The drawing under review shows one solid part. Ordinate dimensions are in mm from its lowest x, y, z. Coordinates: 2 decimals unless noted, no trailing zeros. Write each loop counter-clockwise with the first axis right and the second up, starting at its lowest first coordinate (ties: lowest second). Pieces come first, ordered by that corner, then holes.
1) We need section C-C on z = 55. Write out the cut boundary in (x, y), then the cut area to 3 significant figures.
2) We need section B-B on y = 4.1. Give the number of separate pieces and of enclosed holes in the cut face, then the cut area to 3 significant figures.
3) To check wall thickness, follow line 1 along Z through (x, y) = (27, 3.6); line 2 along Z through (x, y) = (52, 3); line 3 along X through (y, z) = (4.85, 52.5). State the ranges of each line that lie inside material, in increasing order.
4) Insertion check: P1, Ø10, axis at x = 12.5, z = 57.5, coming from the -Y side; P2, Ø2, axis at x = 8.5, y = 3.5, coming from the +Z side. Each pin has a flat end and moves straight along its axis. Give the tip position at first contact, or say it passes through.
5) We need section A-A on x = 27. Write out the cut boundary in (y, z).
6) We need section D-D on z = 22.5. Write out the cut boundary in (x, y), then the cut area to 3 significant figures.
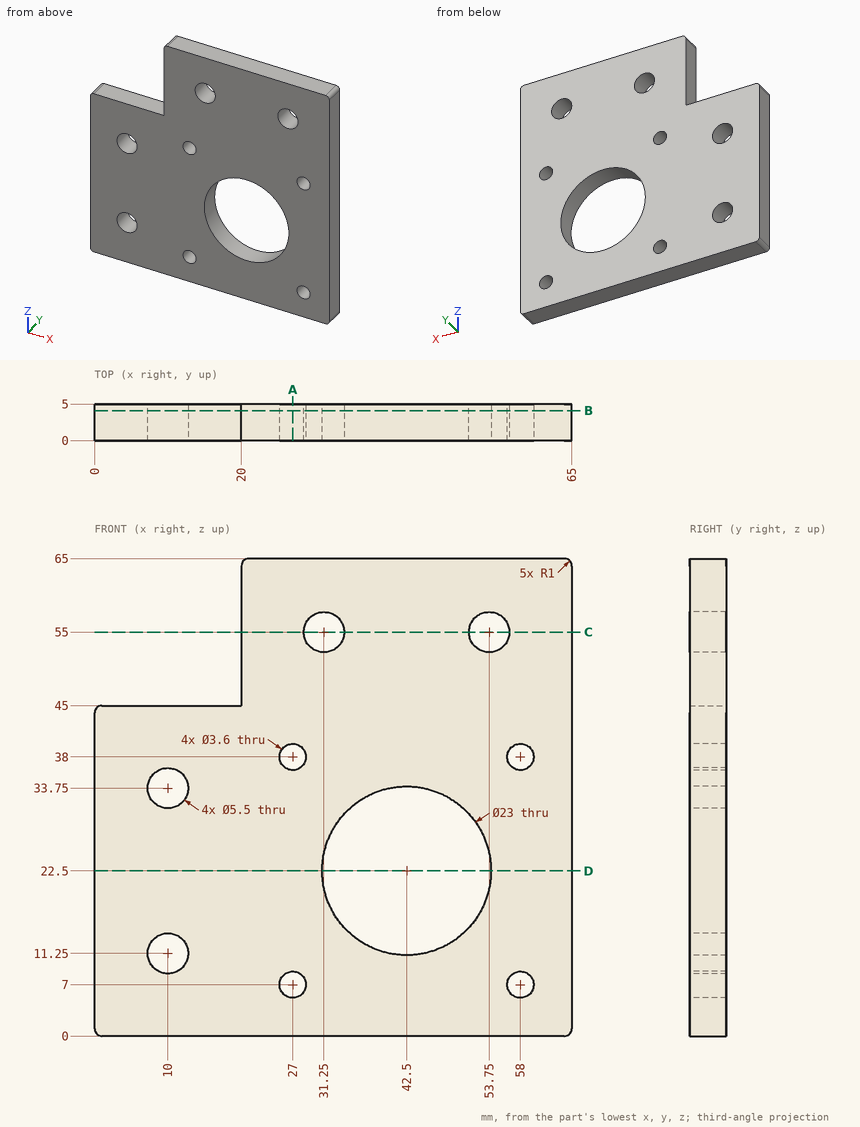
Result:
1. outline: (20, 0) - (28.5, 0) - (28.5, 5) - (20, 5) - close; (34, 0) - (51, 0) - (51, 5) - (34, 5) - close; (56.5, 0) - (65, 0) - (65, 5) - (56.5, 5) - close
1. area: 170 mm2
2. separate pieces: 1
2. enclosed holes: 9
2. area: 3,270 mm2
3. line 1: z = 0 to 5.2, 8.8 to 36.2, 39.8 to 65
3. line 2: z = 0 to 16.02, 28.98 to 52.88, 57.12 to 65
3. line 3: x = 20 to 30.1, 32.4 to 52.6, 54.9 to 65
4. P1: passes through
4. P2: stops at z = 45
5. outline: (0, 0) - (5, 0) - (5, 5.2) - (0, 5.2) - close; (0, 8.8) - (5, 8.8) - (5, 36.2) - (0, 36.2) - close; (0, 39.8) - (5, 39.8) - (5, 65) - (0, 65) - close
6. outline: (0, 0) - (31, 0) - (31, 5) - (0, 5) - close; (54, 0) - (65, 0) - (65, 5) - (54, 5) - close
6. area: 210 mm2
